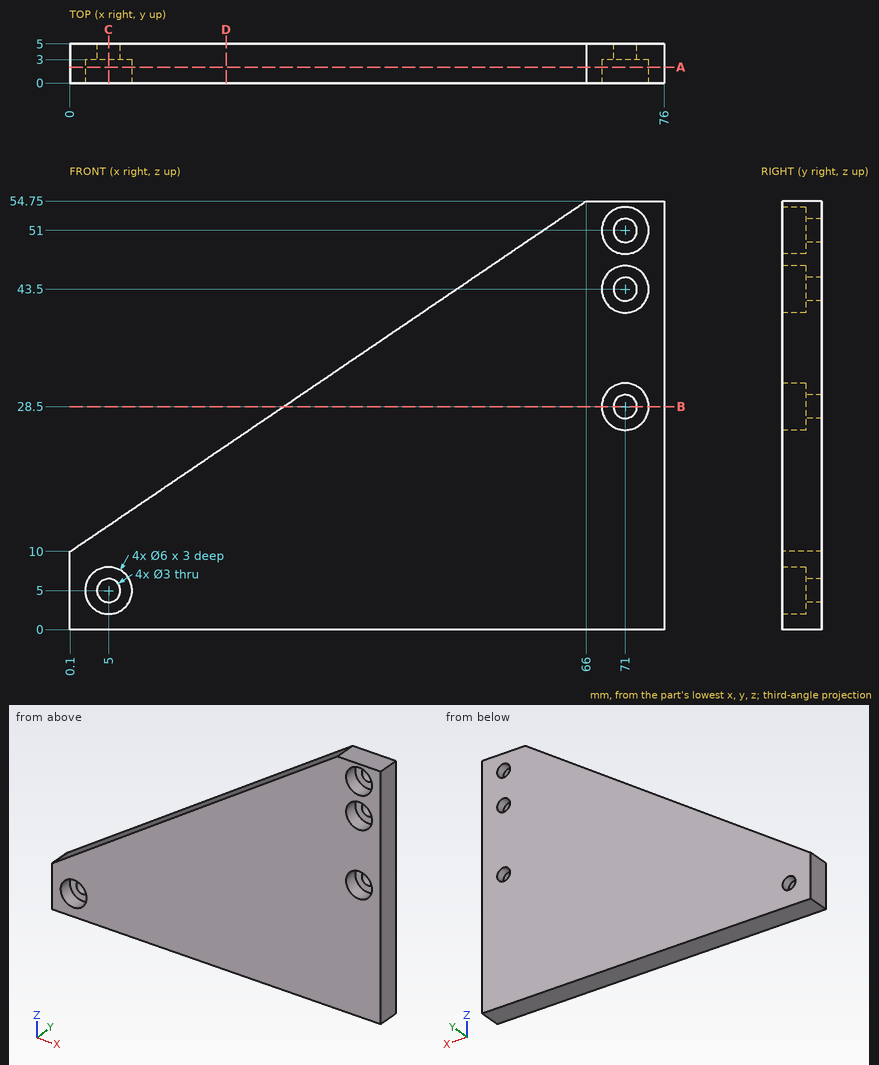
Check sheet for the drawn part. Datum: minimum x, y, z corner. Units: mm. Round coordinates to 2 decimals unless told otherwise and drop trailing zeros. Loops run counter-clockwise (first coordinate to the right, second up) from the corner with the lowest first, then second, coordinate; pieces in that order, holes last.
Item 1: Gauge pin test, flat ends, axial feed: pin 1 (1 mm diameter, centred on x = 48.5, y = 3.5, fed in from -Z); pin 2 (5.5 mm diameter, centred on x = 71, z = 28.5, fed in from -Y); pin 3 (1 mm diameter, centred on x = 39, y = 4.5, fed in from +Z); pin 4 (1 mm diameter, centred on x = 48, y = 0.5, fed in from +Z). Record the tip position at first contact, or that the pin passes through.
Item 2: Thickness scan on line 1 (Z direction, x = 71, y = 3.6); line 2 (Z direction, x = 71, y = 2.2); line 3 (Z direction, x = 5, y = 0.75). Record the ranges inside material, lowest first.
Item 3: Cross-section at C-C on x = 5. Record the boundary of the cut face in (y, z), then the cut area to 3 significant figures.
Item 4: Cross-section at A-A on y = 2.05. Record the boundary of the cut face in (x, z).
Item 5: Cross-section at B-B on z = 28.5. Record the boundary of the cut face in (x, y), then the cut area to 3 significant figures.
Item 6: Cross-section at D-D on x = 20. Record the boundary of the cut face in (y, z).
Answer sheet:
1. pin 1: stops at z = 0
1. pin 2: stops at y = 3
1. pin 3: stops at z = 36.75
1. pin 4: stops at z = 42.87
2. line 1: z = 0 to 27, 30 to 42, 45 to 49.5, 52.5 to 54.75
2. line 2: z = 0 to 25.5, 31.5 to 40.5, 46.5 to 48, 54 to 54.75
2. line 3: z = 0 to 2, 8 to 13.33
3. outline: (0, 0) - (5, 0) - (5, 3.5) - (3, 3.5) - (3, 2) - (0, 2) - close; (0, 8) - (3, 8) - (3, 6.5) - (5, 6.5) - (5, 13.33) - (0, 13.33) - close
3. area: 42.6 mm2
4. outline: (0, 0) - (76, 0) - (76, 54.75) - (66, 54.75) - (0.1, 10) - (0, 10) - close; hole circle Ø6 at (5, 5); hole circle Ø6 at (71, 28.5); hole circle Ø6 at (71, 43.5); hole circle Ø6 at (71, 51)
5. outline: (27.34, 0) - (68, 0) - (68, 3) - (69.5, 3) - (69.5, 5) - (27.34, 5) - close; (72.5, 3) - (74, 3) - (74, 0) - (76, 0) - (76, 5) - (72.5, 5) - close
5. area: 219 mm2
6. outline: (0, 0) - (5, 0) - (5, 23.51) - (0, 23.51) - close
